Geometry check sheet. Reference: the model listing, model coordinates, mm. Face numbers are marked on the shaded views. A direction names the side the tool comes from. Round coordinates to 2 decimals unless told otherwise and drop trailing zeros. Write each loop counter-clockwise with the first axis right and the second up, starting at its lowest first coordinate (ties: lowest second). Pieces come first, ordered by that corner, then holes. Notation, with made-up numbers: (83, -31.75) -> (135, -31.75) arc R18 cw to (135, -2.75) -> close; hole circle Ø10 at (-38.5, -4). An arc over 180 degrees is marked (long way). Put each result on its own line as item: value. Start each with the question number.
from build123d import *

# Parameters (mm, degrees)
SKETCH1_W            = 120
SKETCH1_H            = 80
BOSS_EXTRUDE1_DEPTH  = 60
SHELL3_T             = -6
SKETCH2_W            = 4.722426826
SKETCH2_H            = 30
BOSS_EXTRUDE2_DEPTH  = 15
SKETCH3_W            = 5
SKETCH3_H            = 30
BOSS_EXTRUDE3_DEPTH  = 15
SKETCH4_R            = 2.5
CUT_EXTRUDE2_DEPTH   = 5
CUT_EXTRUDE3_REACH   = 155.052
CUT_EXTRUDE4_DEPTH   = 6
SKETCH7_R            = 2.16
CUT_EXTRUDE5_DEPTH   = 6
SKETCH9_W            = 108
SKETCH9_H            = 68
BOSS_EXTRUDE4_DEPTH  = 10
SKETCH12_R           = 2.16
CUT_EXTRUDE6_DEPTH   = 10
SKETCH13_W           = 120
SKETCH13_H           = 80
CUT_EXTRUDE7_DEPTH   = 10
CUT_EXTRUDE8_REACH   = 122.52
CUT_EXTRUDE9_START   = -44
SKETCH17_W           = 114
SKETCH17_H           = 74
SKETCH17_W_2         = 108
SKETCH17_H_2         = 68
CUT_EXTRUDE9_DEPTH   = 44
BOSS_EXTRUDE5_DEPTH  = 10
SKETCH24_W           = 8.396994042
SKETCH24_H           = 18.728288782
BOSS_EXTRUDE6_DEPTH  = 5
SKETCH28_W           = 3
SKETCH28_H           = 13.054996367
BOSS_EXTRUDE8_DEPTH  = 24
SKETCH29_R           = 1.25
CUT_EXTRUDE10_DEPTH  = 48
SKETCH30_R           = 6
SKETCH30_R_2         = 3
BOSS_EXTRUDE9_DEPTH  = 10
SKETCH31_R           = 6
SKETCH31_R_2         = 1.5
BOSS_EXTRUDE10_DEPTH = 2


with BuildPart() as part:
    # Sketch1 → Boss-Extrude1 (new body)
    with BuildSketch(Plane.XY):
        Rectangle(SKETCH1_W, SKETCH1_H)
    extrude(amount=BOSS_EXTRUDE1_DEPTH)

    # Shell3
    shell3_openings = [part.faces().sort_by_distance(p)[0] for p in [
        (0, 0, 0),
    ]]
    offset(amount=SHELL3_T, openings=shell3_openings, kind=Kind.INTERSECTION)

    # Sketch2 → Boss-Extrude2 (add)
    with BuildSketch(Plane(origin=(60, 0, 0), x_dir=(0, 0, -1), z_dir=(1, 0, 0))):
        with Locations((-2.361213413, 0)):
            Rectangle(SKETCH2_W, SKETCH2_H)
    extrude(amount=BOSS_EXTRUDE2_DEPTH)

    # Sketch3 → Boss-Extrude3 (add)
    with BuildSketch(Plane.ZY.offset(60)):
        with Locations((2.5, 0)):
            Rectangle(SKETCH3_W, SKETCH3_H)
    extrude(amount=BOSS_EXTRUDE3_DEPTH)

    # Sketch4 → Cut-Extrude2 (cut)
    with BuildSketch(Plane.XY.offset(5)):
        with Locations((-67.5, 7.5)):
            Circle(SKETCH4_R)
        with Locations((-67.5, -7.5)):
            Circle(SKETCH4_R)
        with Locations((67.5, -7.5)):
            Circle(SKETCH4_R)
        with Locations((67.5, 7.5)):
            Circle(SKETCH4_R)
    extrude(amount=-CUT_EXTRUDE2_DEPTH, mode=Mode.SUBTRACT)

    # Cut-Extrude3: up to this face of the body (flat: up to its plane)
    cut_extrude3_end = Plane(part.part.faces().sort_by_distance((-60, 0, 30.887096774))[0])
    # Sketch5 → Cut-Extrude3 (cut, up to the picked face)
    with BuildSketch(Plane(origin=(60, 0, 0), x_dir=(0, 0, -1), z_dir=(1, 0, 0)), mode=Mode.PRIVATE) as cut_extrude3_sk1:
        with BuildLine():
            Line((-38, 31.802865199), (-22, 31.802865199))
            ThreePointArc((-22, 31.802865199), (-20.585786438, 31.217078762), (-20, 29.802865199))
            Line((-20, 29.802865199), (-20, 18.802865199))
            ThreePointArc((-20, 18.802865199), (-20.585786438, 17.388651637), (-22, 16.802865199))
            Line((-22, 16.802865199), (-38, 16.802865199))
            ThreePointArc((-38, 16.802865199), (-39.414213562, 17.388651637), (-40, 18.802865199))
            Line((-40, 18.802865199), (-40, 29.802865199))
            ThreePointArc((-40, 29.802865199), (-39.414213562, 31.217078762), (-38, 31.802865199))
        make_face()
    cut_extrude3_tool1 = split(extrude(cut_extrude3_sk1.sketch, amount=-CUT_EXTRUDE3_REACH, mode=Mode.PRIVATE), bisect_by=cut_extrude3_end, keep=Keep.BOTH, mode=Mode.PRIVATE)
    # Sketch5 → Cut-Extrude3 (cut, up to the picked face)
    with BuildSketch(Plane(origin=(60, 0, 0), x_dir=(0, 0, -1), z_dir=(1, 0, 0)), mode=Mode.PRIVATE) as cut_extrude3_sk2:
        with BuildLine():
            Line((-20, -29.802865199), (-20, -18.802865199))
            ThreePointArc((-20, -18.802865199), (-20.585786438, -17.388651637), (-22, -16.802865199))
            Line((-22, -16.802865199), (-38, -16.802865199))
            ThreePointArc((-38, -16.802865199), (-39.414213562, -17.388651637), (-40, -18.802865199))
            Line((-40, -18.802865199), (-40, -29.802865199))
            ThreePointArc((-40, -29.802865199), (-39.414213562, -31.217078762), (-38, -31.802865199))
            Line((-38, -31.802865199), (-22, -31.802865199))
            ThreePointArc((-22, -31.802865199), (-20.585786438, -31.217078762), (-20, -29.802865199))
        make_face()
    cut_extrude3_tool2 = split(extrude(cut_extrude3_sk2.sketch, amount=-CUT_EXTRUDE3_REACH, mode=Mode.PRIVATE), bisect_by=cut_extrude3_end, keep=Keep.BOTH, mode=Mode.PRIVATE)
    add(cut_extrude3_tool1.solids().sort_by(Axis((60, 24.302865, 30), (-1, 0, 0)))[0], mode=Mode.SUBTRACT)
    add(cut_extrude3_tool2.solids().sort_by(Axis((60, -24.302865, 30), (-1, 0, 0)))[0], mode=Mode.SUBTRACT)

    # Sketch6 → Cut-Extrude4 (cut)
    with BuildSketch(Plane.XY.offset(60)):
        with BuildLine():
            Line((-34, 24.918850814), (-34, -24.918850814))
            ThreePointArc((-34, -24.918850814), (-40, -30.918850814), (-46, -24.918850814))
            Line((-46, -24.918850814), (-46, 24.918850814))
            ThreePointArc((-46, 24.918850814), (-40, 30.918850814), (-34, 24.918850814))
        make_face()
        with BuildLine():
            Line((34, 24.918850814), (34, -24.918850814))
            ThreePointArc((34, -24.918850814), (40, -30.918850814), (46, -24.918850814))
            Line((46, -24.918850814), (46, 24.918850814))
            ThreePointArc((46, 24.918850814), (40, 30.918850814), (34, 24.918850814))
        make_face()
    extrude(amount=-CUT_EXTRUDE4_DEPTH, mode=Mode.SUBTRACT)

    # Sketch7 → Cut-Extrude5 (cut)
    with BuildSketch(Plane(origin=(0, 0, 54), x_dir=(-1, 0, 0), z_dir=(0, 0, -1))):
        with Locations((-12.965, 0)):
            Circle(SKETCH7_R)
        with Locations((12.965, 0)):
            Circle(SKETCH7_R)
    extrude(amount=-CUT_EXTRUDE5_DEPTH, mode=Mode.SUBTRACT)

    # Sketch9 → Boss-Extrude4 (add)
    with BuildSketch(Plane(origin=(0, 0, 54), x_dir=(-1, 0, 0), z_dir=(0, 0, -1))):
        Rectangle(SKETCH9_W, SKETCH9_H)
    extrude(amount=BOSS_EXTRUDE4_DEPTH)

    # Sketch12 → Cut-Extrude6 (cut)
    with BuildSketch(Plane.XY.offset(54)):
        with Locations(Location((12.965, 0, 0), (0, 0, 180))):
            Circle(SKETCH12_R)
        with Locations(Location((-12.965, 0, 0), (0, 0, 180))):
            Circle(SKETCH12_R)
        with BuildLine():
            Line((46, -24.918850814), (46, 24.918850814))
            ThreePointArc((46, 24.918850814), (40, 30.918850814), (34, 24.918850814))
            Line((34, 24.918850814), (34, -24.918850814))
            ThreePointArc((34, -24.918850814), (40, -30.918850814), (46, -24.918850814))
        make_face()
        with BuildLine():
            Line((-34, -24.918850814), (-34, 24.918850814))
            ThreePointArc((-34, 24.918850814), (-40, 30.918850814), (-46, 24.918850814))
            Line((-46, 24.918850814), (-46, -24.918850814))
            ThreePointArc((-46, -24.918850814), (-40, -30.918850814), (-34, -24.918850814))
        make_face()
    extrude(amount=-CUT_EXTRUDE6_DEPTH, mode=Mode.SUBTRACT)

    # Sketch13 → Cut-Extrude7 (cut)
    with BuildSketch(Plane.XY.offset(60)):
        Rectangle(SKETCH13_W, SKETCH13_H)
    extrude(amount=-CUT_EXTRUDE7_DEPTH, mode=Mode.SUBTRACT)

    # Cut-Extrude8: up to this face of the body (flat: up to its plane)
    cut_extrude8_end = Plane(part.part.faces().sort_by_distance((0, -40, 25))[0])
    # Sketch14 → Cut-Extrude8 (cut, up to the picked face)
    with BuildSketch(Plane(origin=(0, 40, 0), x_dir=(1, 0, 0), z_dir=(0, 1, 0)), mode=Mode.PRIVATE) as cut_extrude8_sk1:
        with BuildLine():
            Line((-35.763165519, -10), (35.763165519, -10))
            ThreePointArc((35.763165519, -10), (40.763165519, -15), (35.763165519, -20))
            Line((35.763165519, -20), (-35.763165519, -20))
            ThreePointArc((-35.763165519, -20), (-40.763165519, -15), (-35.763165519, -10))
        make_face()
    cut_extrude8_tool1 = split(extrude(cut_extrude8_sk1.sketch, amount=-CUT_EXTRUDE8_REACH, mode=Mode.PRIVATE), bisect_by=cut_extrude8_end, keep=Keep.BOTH, mode=Mode.PRIVATE)
    add(cut_extrude8_tool1.solids().sort_by(Axis((0, 40, 15), (0, -1, 0)))[0], mode=Mode.SUBTRACT)

    # Sketch17 → Cut-Extrude9 (cut)
    with BuildSketch(Plane(origin=(0, 0, 0), x_dir=(-1, 0, 0), z_dir=(0, 0, -1)).offset(CUT_EXTRUDE9_START)):
        Rectangle(SKETCH17_W, SKETCH17_H)
        Rectangle(SKETCH17_W_2, SKETCH17_H_2, mode=Mode.SUBTRACT)
    extrude(amount=CUT_EXTRUDE9_DEPTH, mode=Mode.SUBTRACT)

    # Sketch23 → Boss-Extrude5 (add)
    with BuildSketch(Plane(origin=(0, 0, 44), x_dir=(-1, 0, 0), z_dir=(0, 0, -1))):
        Polygon((-17.15, 14.35), (-17.15, 5), (-14.15, 5), (-14.15, 11.35), (14.15, 11.35), (14.15, 5), (17.15, 5), (17.15, 14.35), align=None)
    extrude(amount=BOSS_EXTRUDE5_DEPTH)

    # Sketch24 → Boss-Extrude6 (add)
    with BuildSketch(Plane(origin=(0, 0, 44), x_dir=(-1, 0, 0), z_dir=(0, 0, -1))):
        Rectangle(SKETCH24_W, SKETCH24_H)
    extrude(amount=BOSS_EXTRUDE6_DEPTH)

    # Sketch28 → Boss-Extrude8 (add)
    with BuildSketch(Plane(origin=(0, 0, 44), x_dir=(-1, 0, 0), z_dir=(0, 0, -1))):
        with Locations((-15.65, -30.472501816)):
            Rectangle(SKETCH28_W, SKETCH28_H)
        with Locations((15.65, -30.472501816)):
            Rectangle(SKETCH28_W, SKETCH28_H)
    extrude(amount=BOSS_EXTRUDE8_DEPTH)

    # Sketch29 → Cut-Extrude10 (cut)
    with BuildSketch(Plane.ZY.offset(17.15)):
        with Locations((26, -28)):
            Circle(SKETCH29_R)
    extrude(amount=-CUT_EXTRUDE10_DEPTH, mode=Mode.SUBTRACT)

    # Sketch30 → Boss-Extrude9 (add)
    # profile 1 of 2: a face of its own
    with BuildSketch(Plane(origin=(0, 0, 44), x_dir=(-1, 0, 0), z_dir=(0, 0, -1))):
        with Locations((-25.4, -4.36)):
            Circle(SKETCH30_R)
        with Locations((-25.4, -4.36)):
            Circle(SKETCH30_R_2, mode=Mode.SUBTRACT)
    # profile 2 of 2: a face of its own
    with BuildSketch(Plane(origin=(0, 0, 44), x_dir=(-1, 0, 0), z_dir=(0, 0, -1))):
        with Locations((25.4, 4.36)):
            Circle(SKETCH30_R)
        with Locations((25.4, 4.36)):
            Circle(SKETCH30_R_2, mode=Mode.SUBTRACT)
    extrude(amount=BOSS_EXTRUDE9_DEPTH)

    # Sketch31 → Boss-Extrude10 (add)
    # profile 1 of 2: a face of its own
    with BuildSketch(Plane(origin=(0, 0, 34), x_dir=(-1, 0, 0), z_dir=(0, 0, -1))):
        with Locations((-25.4, -4.36)):
            Circle(SKETCH31_R)
        with Locations((-25.4, -4.36)):
            Circle(SKETCH31_R_2, mode=Mode.SUBTRACT)
    # profile 2 of 2: a face of its own
    with BuildSketch(Plane(origin=(0, 0, 34), x_dir=(-1, 0, 0), z_dir=(0, 0, -1))):
        with Locations((25.4, 4.36)):
            Circle(SKETCH31_R)
        with Locations((25.4, 4.36)):
            Circle(SKETCH31_R_2, mode=Mode.SUBTRACT)
    extrude(amount=BOSS_EXTRUDE10_DEPTH)


solid = part.part
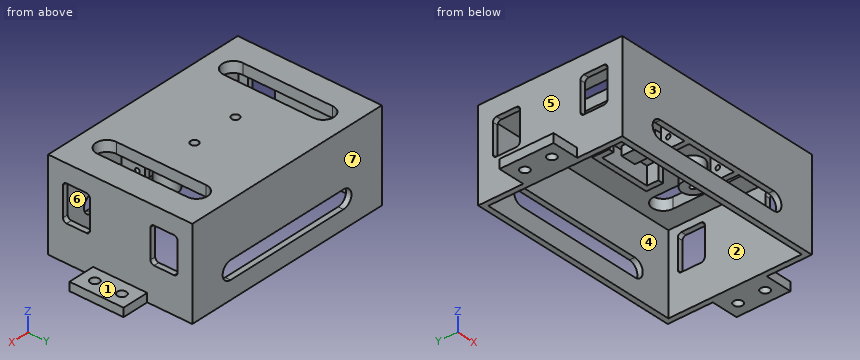
(1) Sectioned sample at B-B (x = 1). Record the cut outline in (y, z), and give its area (3 significant figures).
(2) Material ranges on L1, parallel to Y at x = 67.5, z = 3.5; L2, parallel to Y at x = 15, z = 43.5 (3 decimals); L3, parallel to X at y = 24, z = 48, recorded low to high. Write a range as from..to.
(3) Sectioned sample at A-A (z = 42). State how many separate pieces and enclosed holes the cut face has, and give its area (3 significant figures).
(4) Sectioned sample at D-D (z = 15). Record the cut outline in (x, y).
(5) Go/stop test with flat-tipped pins: pin 1 Ø5 at (y, z) = (7.5, 39.5) entering from +X; pin 2 Ø12 at (y, z) = (26.5, 15) entering from -X; pin 3 Ø8 at (x, y) = (67.5, -7.5) entering from +Z. Record where each tip stops, or that it passes through.
(6) Mould release check, pull along Y, two halves, no side actions. Record for the marked faces 4, 5, 6 and 7: +Y half, -Y half, draft (parallel to the pull), parting line (faces both ways), or undercut.
(7) Set-up check for the marked faces 1, 2 and 3: record each of +Z, -Z, +X, -X, +Y, -Y from which the full face is reachable in a straight line by a thin tool's end or side.
(8) Sectioned sample at C-C (y = -22.5). Record the cut outline in (x, z).
Found:
1. outline: (-40, 0) -> (-37, 0) -> (-37, 10) -> (-40, 10) -> close; (-40, 20) -> (-37, 20) -> (-37, 44) -> (-9.36, 44) -> (-9.36, 39) -> (9.36, 39) -> (9.36, 44) -> (11.35, 44) -> (11.35, 34) -> (14.35, 34) -> (14.35, 44) -> (37, 44) -> (37, 20) -> (40, 20) -> (40, 50) -> (-40, 50) -> close; (37, 0) -> (40, 0) -> (40, 10) -> (37, 10) -> close
1. area: 808 mm2
2. L1: -15..-10, -5..5, 10..15
2. L2: -40..-23.945, 5..14.35, 37..40
2. L3: -60..-46, -34..34, 46..60
3. separate pieces: 5
3. enclosed holes: 3
3. area: 1,710 mm2
4. outline: (-60, -40) -> (-40.76, -40) -> (-40.76, -37) -> (-57, -37) -> (-57, 37) -> (-40.76, 37) -> (-40.76, 40) -> (-60, 40) -> close; (40.76, -40) -> (60, -40) -> (60, 40) -> (40.76, 40) -> (40.76, 37) -> (57, 37) -> (57, -37) -> (40.76, -37) -> close
5. pin 1: x = 60
5. pin 2: x = -60
5. pin 3: z = 4.72
6. face 4: undercut
6. face 5: draft
6. face 6: undercut
6. face 7: +Y half
7. face 1: +Z, +X, +Y, -Y
7. face 2: -Z
7. face 3: +Z, -Z, +X, -X, -Y
8. outline: (-60, 0) -> (-57, 0) -> (-57, 20) -> (-60, 20) -> close; (-60, 40) -> (-57, 40) -> (-57, 44) -> (-46, 44) -> (-46, 50) -> (-60, 50) -> close; (-34, 44) -> (34, 44) -> (34, 50) -> (-34, 50) -> close; (46, 44) -> (57, 44) -> (57, 40) -> (60, 40) -> (60, 50) -> (46, 50) -> close; (57, 0) -> (60, 0) -> (60, 20) -> (57, 20) -> close
